```python
from build123d import *

# Parameters (mm, degrees)
SKETCH1_R             = 1.05
BOSS_EXTRUDE1_DEPTH   = 2.5
SKETCH1_R_2           = 0.95
BOSS_EXTRUDE1_2_DEPTH = 2.5
BOSS_EXTRUDE1_3_DEPTH = 2.5
SKETCH2_R             = 0.95
BOSS_EXTRUDE2_DEPTH   = 9.75
BOSS_EXTRUDE3_START   = -1
SKETCH3_R             = 0.95
SKETCH3_R_2           = 2.75
BOSS_EXTRUDE3_DEPTH   = 1
SKETCH4_R             = 1.75
SKETCH4_R_2           = 0.95
BOSS_EXTRUDE4_DEPTH   = 1
CUT_EXTRUDE3_DEPTH    = 2


with BuildPart() as part:
    # Sketch1 → Boss-Extrude1 (new body)
    with BuildSketch(Plane(origin=(0, 0, 0), x_dir=(1, 0, 0), z_dir=(0, 1, 0))):
        with BuildLine():
            Line((-44.9437148, 2.25), (-11.215142775, 2.25))
            ThreePointArc((-11.215142775, 2.25), (-11.75, 0), (-11.215142775, -2.25))
            Line((-11.215142775, -2.25), (-44.9437148, -2.25))
            ThreePointArc((-44.9437148, -2.25), (-45, 0), (-44.9437148, 2.25))
        make_face()
        with Locations(Location((-42.75, 0, 0), (0, 0, 270))):
            Circle(SKETCH1_R, mode=Mode.SUBTRACT)
    extrude(amount=BOSS_EXTRUDE1_DEPTH)



with BuildPart() as body_2:
    # Sketch1 → Boss-Extrude1 2 (new body)
    with BuildSketch(Plane(origin=(0, 0, 0), x_dir=(1, 0, 0), z_dir=(0, 1, 0))):
        with BuildLine():
            Line((2.25, 44.9437148), (2.25, 5))
            Line((2.25, 5), (6.75, 5))
            ThreePointArc((6.75, 5), (1.75, 0), (6.75, -5))
            Line((6.75, -5), (2.25, -5))
            Line((2.25, -5), (2.25, -44.9437148))
            ThreePointArc((2.25, -44.9437148), (0, -45), (-2.25, -44.9437148))
            Line((-2.25, -44.9437148), (-2.25, -5))
            Line((-2.25, -5), (-6.75, -5))
            ThreePointArc((-6.75, -5), (-1.75, 0), (-6.75, 5))
            Line((-6.75, 5), (-2.25, 5))
            Line((-2.25, 5), (-2.25, 44.9437148))
            ThreePointArc((-2.25, 44.9437148), (0, 45), (2.25, 44.9437148))
        make_face()
        with Locations(Location((0, 0, 0), (0, 0, 270))):
            Circle(SKETCH1_R_2, mode=Mode.SUBTRACT)
        with Locations(Location((0, 42.75, 0), (0, 0, 270))):
            Circle(SKETCH1_R, mode=Mode.SUBTRACT)
        with Locations(Location((0, -42.75, 0), (0, 0, 270))):
            Circle(SKETCH1_R, mode=Mode.SUBTRACT)
    extrude(amount=BOSS_EXTRUDE1_2_DEPTH)


with BuildPart() as body_3:
    # Sketch1 → Boss-Extrude1 3 (new body)
    with BuildSketch(Plane(origin=(0, 0, 0), x_dir=(1, 0, 0), z_dir=(0, 1, 0))):
        with BuildLine():
            Line((44.9437148, -2.25), (11.215142775, -2.25))
            ThreePointArc((11.215142775, -2.25), (11.75, 0), (11.215142775, 2.25))
            Line((11.215142775, 2.25), (44.9437148, 2.25))
            ThreePointArc((44.9437148, 2.25), (45, 0), (44.9437148, -2.25))
        make_face()
        with Locations(Location((42.75, 0, 0), (0, 0, 270))):
            Circle(SKETCH1_R, mode=Mode.SUBTRACT)
    extrude(amount=BOSS_EXTRUDE1_3_DEPTH)


with BuildPart() as part_1:
    add(part.part)

    add(body_2.part)  # Boss-Extrude2 merges body 2

    add(body_3.part)  # Boss-Extrude2 merges body 3
    # Sketch2 → Boss-Extrude2 (add)
    with BuildSketch(Plane(origin=(0, 0, 0), x_dir=(1, 0, 0), z_dir=(0, 1, 0))):
        with BuildLine():
            Line((-6.75, 5), (6.75, 5))
            ThreePointArc((6.75, 5), (11.75, 0), (6.75, -5))
            Line((6.75, -5), (-6.75, -5))
            ThreePointArc((-6.75, -5), (-11.75, 0), (-6.75, 5))
        make_face()
        with Locations(Location((0, 0, 0), (0, 0, 270))):
            Circle(SKETCH2_R, mode=Mode.SUBTRACT)
        with BuildLine():
            Line((-7, 3.992179856), (-7, 3.492179856))
            Line((-7, 3.492179856), (-6.5, 3.492179856))
            Line((-6.5, 3.492179856), (-6.5, 3.992179856))
            ThreePointArc((-6.5, 3.992179856), (-3.921572875, 2.828427125), (-2.757820144, 0.25))
            Line((-2.757820144, 0.25), (-3.257820144, 0.25))
            Line((-3.257820144, 0.25), (-3.257820144, -0.25))
            Line((-3.257820144, -0.25), (-2.757820144, -0.25))
            ThreePointArc((-2.757820144, -0.25), (-3.921572875, -2.828427125), (-6.5, -3.992179856))
            Line((-6.5, -3.992179856), (-6.5, -3.492179856))
            Line((-6.5, -3.492179856), (-7, -3.492179856))
            Line((-7, -3.492179856), (-7, -3.992179856))
            ThreePointArc((-7, -3.992179856), (-9.578427125, -2.828427125), (-10.742179856, -0.25))
            Line((-10.742179856, -0.25), (-10.242179856, -0.25))
            Line((-10.242179856, -0.25), (-10.242179856, 0.25))
            Line((-10.242179856, 0.25), (-10.742179856, 0.25))
            ThreePointArc((-10.742179856, 0.25), (-9.578427125, 2.828427125), (-7, 3.992179856))
        make_face(mode=Mode.SUBTRACT)
        with BuildLine():
            Line((6.5, 3.992179856), (6.5, 3.492179856))
            Line((6.5, 3.492179856), (7, 3.492179856))
            Line((7, 3.492179856), (7, 3.992179856))
            ThreePointArc((7, 3.992179856), (9.578427125, 2.828427125), (10.742179856, 0.25))
            Line((10.742179856, 0.25), (10.242179856, 0.25))
            Line((10.242179856, 0.25), (10.242179856, -0.25))
            Line((10.242179856, -0.25), (10.742179856, -0.25))
            ThreePointArc((10.742179856, -0.25), (9.578427125, -2.828427125), (7, -3.992179856))
            Line((7, -3.992179856), (7, -3.492179856))
            Line((7, -3.492179856), (6.5, -3.492179856))
            Line((6.5, -3.492179856), (6.5, -3.992179856))
            ThreePointArc((6.5, -3.992179856), (3.921572875, -2.828427125), (2.757820144, -0.25))
            Line((2.757820144, -0.25), (3.257820144, -0.25))
            Line((3.257820144, -0.25), (3.257820144, 0.25))
            Line((3.257820144, 0.25), (2.757820144, 0.25))
            ThreePointArc((2.757820144, 0.25), (3.921572875, 2.828427125), (6.5, 3.992179856))
        make_face(mode=Mode.SUBTRACT)
        with BuildLine():
            Line((-3.75, 4), (3.75, 4))
            ThreePointArc((3.75, 4), (2.479758346, 2.600968322), (1.819444444, 0.830434774))
            ThreePointArc((1.819444444, 0.830434774), (0, 2), (-1.819444444, 0.830434774))
            ThreePointArc((-1.819444444, 0.830434774), (-2.479758346, 2.600968322), (-3.75, 4))
        make_face(mode=Mode.SUBTRACT)
        with BuildLine():
            Line((-3.75, -4), (3.75, -4))
            ThreePointArc((3.75, -4), (2.479758346, -2.600968322), (1.819444444, -0.830434774))
            ThreePointArc((1.819444444, -0.830434774), (0, -2), (-1.819444444, -0.830434774))
            ThreePointArc((-1.819444444, -0.830434774), (-2.479758346, -2.600968322), (-3.75, -4))
        make_face(mode=Mode.SUBTRACT)
    extrude(amount=BOSS_EXTRUDE2_DEPTH)

    # Sketch3 → Boss-Extrude3 (add)
    with BuildSketch(Plane(origin=(0, 9.75, 0), x_dir=(1, 0, 0), z_dir=(0, 1, 0)).offset(BOSS_EXTRUDE3_START)):
        with BuildLine():
            Line((-6.75, 5), (6.75, 5))
            ThreePointArc((6.75, 5), (11.75, 0), (6.75, -5))
            Line((6.75, -5), (-6.75, -5))
            ThreePointArc((-6.75, -5), (-11.75, 0), (-6.75, 5))
        make_face()
        with Locations(Location((0, 0, 0), (0, 0, 270))):
            Circle(SKETCH3_R, mode=Mode.SUBTRACT)
        with Locations(Location((-6.75, 0, 0), (0, 0, 270))):
            Circle(SKETCH3_R_2, mode=Mode.SUBTRACT)
        with Locations(Location((6.75, 0, 0), (0, 0, 270))):
            Circle(SKETCH3_R_2, mode=Mode.SUBTRACT)
    extrude(amount=BOSS_EXTRUDE3_DEPTH)

    # Sketch4 → Boss-Extrude4 (add)
    with BuildSketch(Plane(origin=(0, 9.75, 0), x_dir=(1, 0, 0), z_dir=(0, 1, 0))):
        with Locations(Location((0, 0, 0), (0, 0, 270))):
            Circle(SKETCH4_R)
        with Locations(Location((0, 0, 0), (0, 0, 270))):
            Circle(SKETCH4_R_2, mode=Mode.SUBTRACT)
    extrude(amount=BOSS_EXTRUDE4_DEPTH)

    # Sketch7 → Cut-Extrude3 (cut)
    with BuildSketch(Plane(origin=(11.75, 0, 0), x_dir=(0, 0, -1), z_dir=(1, 0, 0))):
        with BuildLine():
            Line((-1, 8.75), (1, 8.75))
            ThreePointArc((1, 8.75), (1.5, 8.25), (1, 7.75))
            Line((1, 7.75), (-1, 7.75))
            ThreePointArc((-1, 7.75), (-1.5, 8.25), (-1, 8.75))
        make_face()
    extrude(amount=-CUT_EXTRUDE3_DEPTH, mode=Mode.SUBTRACT)


solid = part_1.part
```
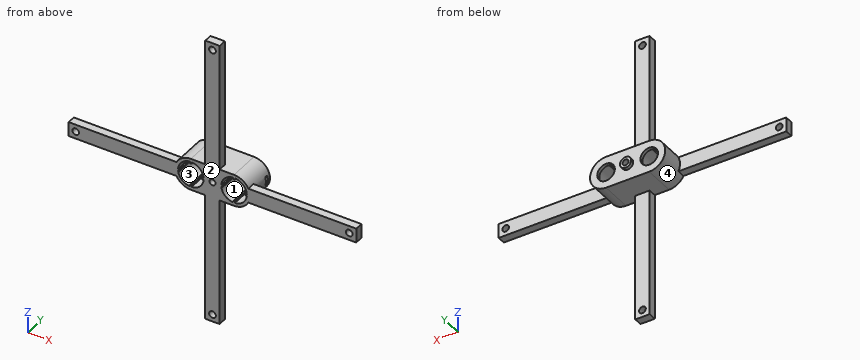
Check sheet for the modelled part. Datum: model origin and axes. Units: mm. Face numbers are marked on the shaded views. Give positions to 0.01 mm unless a question says otherwise; leave off trailing zeros. Order: outer loops, then holes, each group sorted by start corner. A loop starts at its lowest first (then second) coordinate and runs counter-clockwise, first axis right, second up. Notation, with made-up numbers: (55.25, -37) -> (70.25, -37) arc R32 cw to (70.25, -6) -> close; hole circle Ø9 at (13.25, 67.5). An arc over 180 degrees is marked (long way). Use CSV: the item, a comma, the result in double quotes. Start each with the question number.
1) Sectioned sample at C-C, the plane x = 31. Record the boundary of the cut face in (y, z).
2) Mould release check, pull along Z, two halves, no side actions. Record for the marked faces 1, 2, 3 and 4: released by +Z, released by -Z, zero draft, split by the parting line, or undercut.
3) Go/stop test with flat-tipped pins: P1, Ø1, axis at x = 21, y = 1, coming from the +Z side; P2, Ø3, axis at y = 1, z = 17, coming from the +X side; P3, Ø2, axis at y = 2.5, z = 2, coming from the -X side. Record where each tip stops, or that it passes through.
4) Material ranges on line 1 (X direction, y = 9.3, z = 0); line 2 (Z direction, x = -9, y = 3.75); line 3 (X direction, y = 0.75, z = 27.5), recorded low to high. Write a range as from..to.
5) Sectioned sample at B-B, the plane x = -42.75. Record the boundary of the cut face in (y, z), plus the area to 3 significant figures.
6) Sectioned sample at D-D, the plane z = -39. Record the boundary of the cut face in (x, y), plus the area to 4 significant figures.
7) Sectioned sample at A-A, the plane z = 42.75. Record the boundary of the cut face in (x, y), plus the area to 3 significant figures.
Recorded:
1,outline,"(0, -2.25) -> (2.5, -2.25) -> (2.5, 2.25) -> (0, 2.25) -> close"
2,face 1,"undercut"
2,face 2,"zero draft"
2,face 3,"undercut"
2,face 4,"split by the parting line"
3,P1,"z = 2.25"
3,P2,"x = 2.25"
3,P3,"x = -44.99"
4,line 1,"-11.75..-9.5, -4..-0.95, 0.95..4, 9.5..11.75"
4,line 2,"-4.47..-3.31, 3.31..4.47"
4,line 3,"-2.25..2.25"
5,outline,"(0, -2.25) -> (2.5, -2.25) -> (2.5, -1.05) -> (0, -1.05) -> close; (0, 1.05) -> (2.5, 1.05) -> (2.5, 2.25) -> (0, 2.25) -> close"
5,area,"6.00 mm2"
6,outline,"(-2.25, 0) -> (2.25, 0) -> (2.25, 2.5) -> (-2.25, 2.5) -> close"
6,area,"11.25 mm2"
7,outline,"(-2.25, 0) -> (-1.05, 0) -> (-1.05, 2.5) -> (-2.25, 2.5) -> close; (1.05, 0) -> (2.25, 0) -> (2.25, 2.5) -> (1.05, 2.5) -> close"
7,area,"6.00 mm2"
